```python
from build123d import *

# Parameters (mm, degrees)
SKETCH1_R               = 15
BOSS_EXTRUDE1_DEPTH     = 20
SKETCH2_R               = 5
CUT_EXTRUDE1_DEPTH      = 16
CUT_EXTRUDE1_DEPTH_BACK = 16
SKETCH3_W               = 15
SKETCH3_H               = 16
CUT_EXTRUDE2_DEPTH      = 16.0000001
CUT_EXTRUDE2_DEPTH_BACK = 16.0000001
FILLET1_R               = 2


with BuildPart() as part:
    # Sketch1 → Boss-Extrude1 (new body)
    with BuildSketch(Plane(origin=(0, 0, 0), x_dir=(1, 0, 0), z_dir=(0, 1, 0))):
        Circle(SKETCH1_R)
    extrude(amount=BOSS_EXTRUDE1_DEPTH)

    # Sketch2 → Cut-Extrude1 (cut, two sides)
    with BuildSketch(Plane(origin=(0, 0, 0), x_dir=(0, 0, -1), z_dir=(1, 0, 0))) as cut_extrude1_sk:
        with BuildLine():
            ThreePointArc((-15, 10), (-12.071067812, 17.071067812), (-5, 20))
            Line((-5, 20), (-15, 20))
            Line((-15, 20), (-15, 10))
        make_face()
        with BuildLine():
            Line((15, 20), (5, 20))
            ThreePointArc((5, 20), (12.071067812, 17.071067812), (15, 10))
            Line((15, 10), (15, 20))
        make_face()
        with Locations((0, 10)):
            Circle(SKETCH2_R)
    extrude(amount=CUT_EXTRUDE1_DEPTH, mode=Mode.SUBTRACT)
    extrude(cut_extrude1_sk.sketch, amount=-CUT_EXTRUDE1_DEPTH_BACK, mode=Mode.SUBTRACT)

    # Sketch3 → Cut-Extrude2 (cut, two sides)
    with BuildSketch(Plane.XY) as cut_extrude2_sk:
        with Locations((0, 12)):
            Rectangle(SKETCH3_W, SKETCH3_H)
    extrude(amount=CUT_EXTRUDE2_DEPTH, mode=Mode.SUBTRACT)
    extrude(cut_extrude2_sk.sketch, amount=-CUT_EXTRUDE2_DEPTH_BACK, mode=Mode.SUBTRACT)

    # Fillet1
    fillet1_edges = [part.edges().sort_by_distance(p)[0] for p in [
        (7.5, 20, 0),
        (-7.5, 20, 0),
        (7.5, 18.947849992, -9.464972622),
        (7.5, 18.94784999, 9.464972627),
        (-7.5, 18.94784999, -9.464972627),
        (-7.5, 18.947849992, 9.464972622),
    ]]
    fillet(fillet1_edges, radius=FILLET1_R)


solid = part.part
```
Design review of the part built by this model. Coordinates are the model's own, in mm. A direction names the side the tool comes from. Coordinates: 2 decimals unless noted, no trailing zeros. Order: outer loops, then holes, each group sorted by start corner. A loop starts at its lowest first (then second) coordinate and runs counter-clockwise, first axis right, second up. Notation, with made-up numbers: (-38.5, 40) - (5.5, 40) arc R34 ccw to (5.5, 77) - close; hole circle Ø6 at (-18, 61.5). An arc over 180 degrees is marked (long way). Answer in a Markdown table with one row per item.
(1) Consider section C-C on x = -8. State the section outline as (y, z) points.
Checked values:
| item | result |
|---|---|
| outline | (0, -12.69) - (15.27, -12.69) arc R9.32 ccw to (19.32, -5) - (19.32, 5) arc R9.32 ccw to (15.27, 12.69) - (0, 12.69) - close; hole circle Ø10 at (10, 0) |
(2) Clearance check with flat-ended pins moving along their axes: pin 1 (10 mm diameter, centred on x = 9.5, y = 2.5, fed in from -Z); pin 2 (8 mm diameter, centred on x = -9, y = 12.5, fed in from +Z); pin 3 (1.5 mm diameter, centred on x = 9, y = 6, fed in from -Z). State where each tip first meets the part, or that it passes through.
Checked values:
| item | result |
|---|---|
| pin 1 | z = -14.31 |
| pin 2 | z = 12.99 |
| pin 3 | z = -12.53 |
(3) Consider section D-D on z = 4. State the section outline as (x, y) points.
Checked values:
| item | result |
|---|---|
| outline | (-14.46, 0) - (14.46, 0) - (14.46, 7) - (7.5, 7) - (7.5, 4) - (-7.5, 4) - (-7.5, 7) - (-14.46, 7) - close; (-14.46, 13) - (-7.5, 13) - (-7.5, 18) arc R2 ccw to (-9.5, 20) - (-14.46, 20) - close; (7.5, 13) - (14.46, 13) - (14.46, 20) - (9.5, 20) arc R2 ccw to (7.5, 18) - close |
(4) Consider section A-A on z = 0. State the section outline as (x, y) points, plus the area to 3 significant figures.
Checked values:
| item | result |
|---|---|
| outline | (-15, 0) - (15, 0) - (15, 5) - (7.5, 5) - (7.5, 4) - (-7.5, 4) - (-7.5, 5) - (-15, 5) - close; (-15, 15) - (-7.5, 15) - (-7.5, 18) arc R2 ccw to (-9.5, 20) - (-15, 20) - close; (7.5, 15) - (15, 15) - (15, 20) - (9.5, 20) arc R2 ccw to (7.5, 18) - close |
| area | 208 mm^2 |
(5) The part is to be moulded in two halves that separate along Y. For faces 1 (the cylindrical face through (11.198, 14.957, 0.651)), 2 (the cylindrical face through (8.07, 19.4, 0.07)), 3 (the flat face through (7.5, 16, 0)), say which applies: released by +Y, released by -Y, zero draft, split by the parting line, or undercut.
Checked values:
| item | result |
|---|---|
| face 1 | undercut |
| face 2 | released by +Y |
| face 3 | zero draft |
(6) For faces 4 (the cylindrical face through (11.273, 19.622, -7.722)), 5 (the cylindrical face through (-8.1, 19.43, 0.07)), list the 3-axis set-ups (+Z, -Z, +X, -X, +Y, -Y) from which the entire face can be reached by the end or side of a thin tool; tool diameter is ignored.
Checked values:
| item | result |
|---|---|
| face 4 | -Z, +X, -X, +Y |
| face 5 | +Z, -Z, +Y |
(7) Wall thickness on line 1 along Y through (x, z) = (-12.75, 0); line 2 along Y through (x, z) = (-2, 10); line 3 along X through (y, z) = (5, 5): over which ranges is each line inside the solid? List them lowest first. Write a range as from..to.
Checked values:
| item | result |
|---|---|
| line 1 | 0..5, 15..20 |
| line 2 | 0..4 |
| line 3 | -14.14..-7.5, 7.5..14.14 |
(8) Consider section B-B on y = 10. State the section outline as (x, z) points, plus the area to 3 significant figures.
Checked values:
| item | result |
|---|---|
| outline | (-14.14, -5) arc R15 ccw to (-7.5, -12.99) - (-7.5, -5) - close; (-14.14, 5) - (-7.5, 5) - (-7.5, 12.99) arc R15 ccw to start; (7.5, -12.99) arc R15 ccw to (14.14, -5) - (7.5, -5) - close; (7.5, 5) - (14.14, 5) arc R15 ccw to (7.5, 12.99) - close |
| area | 132 mm^2 |
